Can you work these out from the model? Positions are in its coordinate system, mm. Coordinates: 2 decimals unless noted, no trailing zeros. Order: outer loops, then holes, each group sorted by start corner. A loop starts at its lowest first (then second) coordinate and runs counter-clockwise, first axis right, second up. Notation, with made-up numbers: (79.25, 61) -> (133.25, 61) arc R21 ccw to (133.25, 93) -> close; hole circle Ø7 at (76.25, 5). An arc over 180 degrees is marked (long way). Use a Markdown table: item, result. Add a question column.
1. Suppose I cut it at B-B, the plane z = -180.5. List the corners of the cut face in (x, y) for me.
2. If I drill on line 1 along Z through (x, y) = (-304.5, 3.5); line 2 along X through (y, z) = (13, -258.5); line 3 along X through (y, z) = (23.25, -257), over which ranges is the centre line in solid material (lowest first)? Write a range as from..to.
3. Suppose I cut it at C-C, the plane y = 15. List the corners of the cut face in (x, z) for me, then the cut area to 3 significant figures.
4. For pin 1 Ø1.5 at (x, y) = (-211, 5) entering from +Z, with a flat end and sliding along its axis, tell me the tip position at first contact or that it passes through.
5. Suppose I cut it at A-A, the plane x = -242. List the corners of the cut face in (y, z) for me, then the cut area to 3 significant figures.
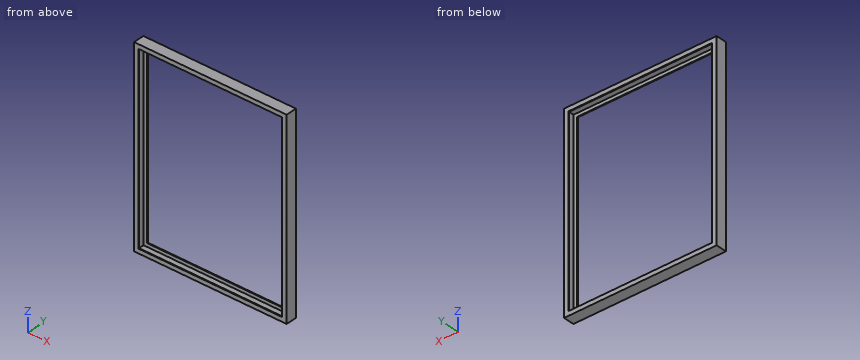
```python
from build123d import *

# Parameters (mm, degrees)
SKETCH1_W           = 350
SKETCH1_H           = 440
SKETCH1_W_2         = 330
SKETCH1_H_2         = 420
BOSS_EXTRUDE1_DEPTH = 25
SHELL1_T            = -2


with BuildPart() as part:
    # Sketch1 → Boss-Extrude1 (new body)
    with BuildSketch(Plane(origin=(0, 0, 0), x_dir=(1, 0, 0), z_dir=(0, 1, 0))):
        with Locations((-175, 220)):
            Rectangle(SKETCH1_W, SKETCH1_H)
        with Locations((-175, 220)):
            Rectangle(SKETCH1_W_2, SKETCH1_H_2, mode=Mode.SUBTRACT)
    extrude(amount=BOSS_EXTRUDE1_DEPTH)

    # Shell1
    shell1_openings = [part.faces().sort_by_distance(p)[0] for p in [
        (-175, 12.5, -10),
        (-10, 12.5, -220),
        (-175, 12.5, -430),
        (-340, 12.5, -220),
    ]]
    offset(amount=SHELL1_T, openings=shell1_openings, kind=Kind.INTERSECTION)


solid = part.part
```
Worked out:
| question | item | result |
|---|---|---|
| 1 | outline | (-350, 0) -> (-340, 0) -> (-340, 2) -> (-348, 2) -> (-348, 23) -> (-340, 23) -> (-340, 25) -> (-350, 25) -> close; (-10, 0) -> (0, 0) -> (0, 25) -> (-10, 25) -> (-10, 23) -> (-2, 23) -> (-2, 2) -> (-10, 2) -> close |
| 2 | line 1 | z = -440..-438, -2..0 |
| 2 | line 2 | x = -350..-348, -2..0 |
| 2 | line 3 | x = -350..-340, -10..0 |
| 3 | outline | (-350, -440) -> (0, -440) -> (0, 0) -> (-350, 0) -> close; hole (-348, -438) -> (-2, -438) -> (-2, -2) -> (-348, -2) -> close |
| 3 | area | 3,140 mm² |
| 4 | pin 1 | stops at z = 0 |
| 5 | outline | (0, -440) -> (25, -440) -> (25, -430) -> (23, -430) -> (23, -438) -> (2, -438) -> (2, -430) -> (0, -430) -> close; (0, -10) -> (2, -10) -> (2, -2) -> (23, -2) -> (23, -10) -> (25, -10) -> (25, 0) -> (0, 0) -> close |
| 5 | area | 164 mm² |
